Drawing for the job (mm, zero at the part's lowest x, y, z). Coordinates: 2 decimals unless noted, no trailing zeros. Order: outer loops, then holes, each group sorted by start corner. A loop starts at its lowest first (then second) coordinate and runs counter-clockwise, first axis right, second up.
1) Cut at A-A (x = 40.5). List the corners of the cut face in (y, z), and give its area (3 significant figures).
2) Cut at D-D (x = 13.5). List the corners of the cut face in (y, z), and give its area (3 significant figures).
3) Cut at B-B (y = 31.5). List the corners of the cut face in (x, z), and give its area (3 significant figures).
4) Pin check, flat tips, straight feed: pin 1 Ø1 at (x, z) = (11, 2) entering from +Y; pin 2 Ø1.5 at (y, z) = (25.5, 1.5) entering from +X. Stop position of each tip, or through.
5) Wall check: L1, parallel to Y at x = 5.5, z = 2.6; L2, parallel to Y at x = 13.5, z = 1.05; L3, parallel to X at y = 30.5, z = 2.8. Give the ranges that are in metal, low to high.
6) Cut at C-C (y = 22.5). List the corners of the cut face in (x, z), and give its area (3 significant figures).
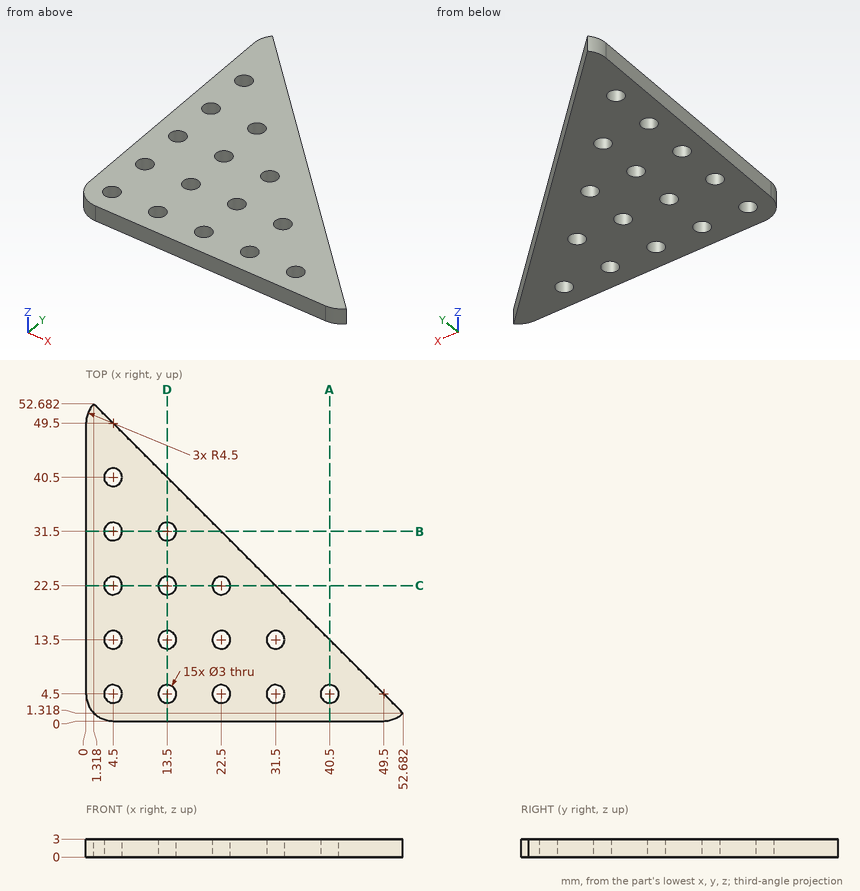
Geometry check:
1. outline: (0, 0) - (3, 0) - (3, 3) - (0, 3) - close; (6, 0) - (13.5, 0) - (13.5, 3) - (6, 3) - close
1. area: 31.5 mm2
2. outline: (0, 0) - (3, 0) - (3, 3) - (0, 3) - close; (6, 0) - (12, 0) - (12, 3) - (6, 3) - close; (15, 0) - (21, 0) - (21, 3) - (15, 3) - close; (24, 0) - (30, 0) - (30, 3) - (24, 3) - close; (33, 0) - (40.5, 0) - (40.5, 3) - (33, 3) - close
2. area: 85.5 mm2
3. outline: (0, 0) - (3, 0) - (3, 3) - (0, 3) - close; (6, 0) - (12, 0) - (12, 3) - (6, 3) - close; (15, 0) - (22.5, 0) - (22.5, 3) - (15, 3) - close
3. area: 49.5 mm2
4. pin 1: stops at y = 43.5
4. pin 2: stops at x = 29.25
5. L1: y = 0 to 3.38, 5.62 to 12.38, 14.62 to 21.38, 23.62 to 30.38, 32.62 to 39.38, 41.62 to 48.5
5. L2: y = 0 to 3, 6 to 12, 15 to 21, 24 to 30, 33 to 40.5
5. L3: x = 0 to 3.38, 5.62 to 12.38, 14.62 to 23.5
6. outline: (0, 0) - (3, 0) - (3, 3) - (0, 3) - close; (6, 0) - (12, 0) - (12, 3) - (6, 3) - close; (15, 0) - (21, 0) - (21, 3) - (15, 3) - close; (24, 0) - (31.5, 0) - (31.5, 3) - (24, 3) - close
6. area: 67.5 mm2
